from build123d import *

# Parameters (mm, degrees)
SKETCH1_R           = 38.5
SKETCH1_R_2         = 1.5
SKETCH1_R_3         = 2
SKETCH1_R_4         = 7.5
BOSS_EXTRUDE1_DEPTH = 3


with BuildPart() as part:
    # Sketch1 → Boss-Extrude1 (new body)
    with BuildSketch(Plane.XY):
        Circle(SKETCH1_R)
        with Locations((0, 11)):
            Circle(SKETCH1_R_2, mode=Mode.SUBTRACT)
        with Locations((0, 35.5)):
            Circle(SKETCH1_R_3, mode=Mode.SUBTRACT)
        with Locations((35.5, 0)):
            Circle(SKETCH1_R_3, mode=Mode.SUBTRACT)
        with Locations((11, 0)):
            Circle(SKETCH1_R_2, mode=Mode.SUBTRACT)
        with Locations((0, -35.5)):
            Circle(SKETCH1_R_3, mode=Mode.SUBTRACT)
        with Locations((0, -11)):
            Circle(SKETCH1_R_2, mode=Mode.SUBTRACT)
        with Locations((-35.5, 0)):
            Circle(SKETCH1_R_3, mode=Mode.SUBTRACT)
        with Locations((-11, 0)):
            Circle(SKETCH1_R_2, mode=Mode.SUBTRACT)
        Circle(SKETCH1_R_4, mode=Mode.SUBTRACT)
    extrude(amount=BOSS_EXTRUDE1_DEPTH)


solid = part.part
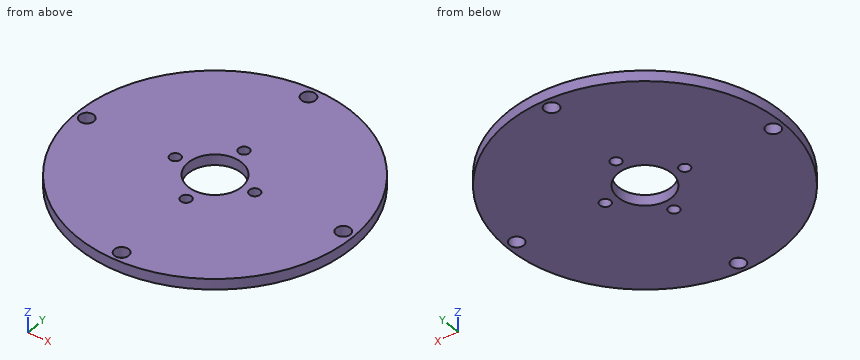
The listing builds one solid part. Answer for the finished solid, in the listing's coordinates (mm). Coordinates: 2 decimals unless noted, no trailing zeros. Loops run counter-clockwise (first coordinate to the right, second up) from the corner with the lowest first, then second, coordinate; pieces in that order, holes last. Notation, with made-up numbers: (-4.75, 9) -> (29.25, 9) arc R30 cw to (29.25, 41) -> close; hole circle Ø11 at (66.5, 58). An arc over 180 degrees is marked (long way). Answer in a Markdown table with one row per item. Add a question column.
1. The part is cut by section A-A, the plane y = 0. Write down the section's boundary in (x, z), then the cut area to 3 significant figures.
2. The part is cut by section B-B, the plane y = 11. Write down the section's boundary in (x, z).
3. A flat-ended cylindrical pin translates along its axis: P1, Ø1, axis at y = 12, z = 0.5, coming from the +X side. Find the tip coordinate at first contact, or state that the pin passes through.
4. Consider line 1 (Y direction, x = 0, z = 1.1); line 2 (Y direction, x = -11, z = 2.35); line 3 (Y direction, x = 6, z = 0.9). Determine where each line is inside the solid, lowest interval first. Write a range as [from, to].
5. The part is cut by section D-D, the plane x = 35.5. Write down the section's boundary in (y, z), then the cut area to 3 significant figures.
6. The part is cut by section C-C, the plane z = 1.8. Count the separate pieces of the cut face and the enclosed holes in it, then the cut area to 3 significant figures.
Answer below:
| question | item | result |
|---|---|---|
| 1 | outline | (-38.5, 0) -> (-37.5, 0) -> (-37.5, 3) -> (-38.5, 3) -> close; (-33.5, 0) -> (-12.5, 0) -> (-12.5, 3) -> (-33.5, 3) -> close; (-9.5, 0) -> (-7.5, 0) -> (-7.5, 3) -> (-9.5, 3) -> close; (7.5, 0) -> (9.5, 0) -> (9.5, 3) -> (7.5, 3) -> close; (12.5, 0) -> (33.5, 0) -> (33.5, 3) -> (12.5, 3) -> close; (37.5, 0) -> (38.5, 0) -> (38.5, 3) -> (37.5, 3) -> close |
| 1 | area | 144 mm2 |
| 2 | outline | (-36.9, 0) -> (-1.5, 0) -> (-1.5, 3) -> (-36.9, 3) -> close; (1.5, 0) -> (36.9, 0) -> (36.9, 3) -> (1.5, 3) -> close |
| 3 | P1 | x = 36.74 |
| 4 | line 1 | [-38.5, -37.5], [-33.5, -12.5], [-9.5, -7.5], [7.5, 9.5], [12.5, 33.5], [37.5, 38.5] |
| 4 | line 2 | [-36.9, -1.5], [1.5, 36.9] |
| 4 | line 3 | [-38.03, -4.5], [4.5, 38.03] |
| 5 | outline | (-14.9, 0) -> (-2, 0) -> (-2, 3) -> (-14.9, 3) -> close; (2, 0) -> (14.9, 0) -> (14.9, 3) -> (2, 3) -> close |
| 5 | area | 77.4 mm2 |
| 6 | separate pieces | 1 |
| 6 | enclosed holes | 9 |
| 6 | area | 4,400 mm2 |
